Verification items for this drawing (mm, ordinates from the low corner). Coordinates: 2 decimals unless noted, no trailing zeros. Write each loop counter-clockwise with the first axis right and the second up, starting at its lowest first coordinate (ties: lowest second). Pieces come first, ordered by that corner, then holes. Notation, with made-up numbers: M 6,50.5 L 33,50.5 A32 ccw 33,78.5 Z; hole C -24,56.5 d6. An arc over 180 degrees is marked long. Put each result on its own line as item: value. Start each with the question number.
1) Cross-section at B-B on z = 0.8. Record the cut outline in (x, y), plus the area to 3 significant figures.
2) Cross-section at D-D on x = 139.5. Record the cut outline in (y, z).
3) Cross-section at C-C on y = 164.5. Record the cut outline in (x, z).
4) Gauge pin test, flat end, axial feed: pin 1 (1 mm diameter, centred on x = 141, z = 2.5, fed in from -Y). Record the tip position at first contact, or that the pin passes through.
5) Scan lines: line 1 along Y through (x, z) = (35, 2.3); line 2 along Y through (x, z) = (60, 0.8); line 3 along Y through (x, z) = (119, 2.1). Record each from-to range of solid material in increasing order.
6) Cross-section at A-A on x = 60. Record the cut outline in (y, z).
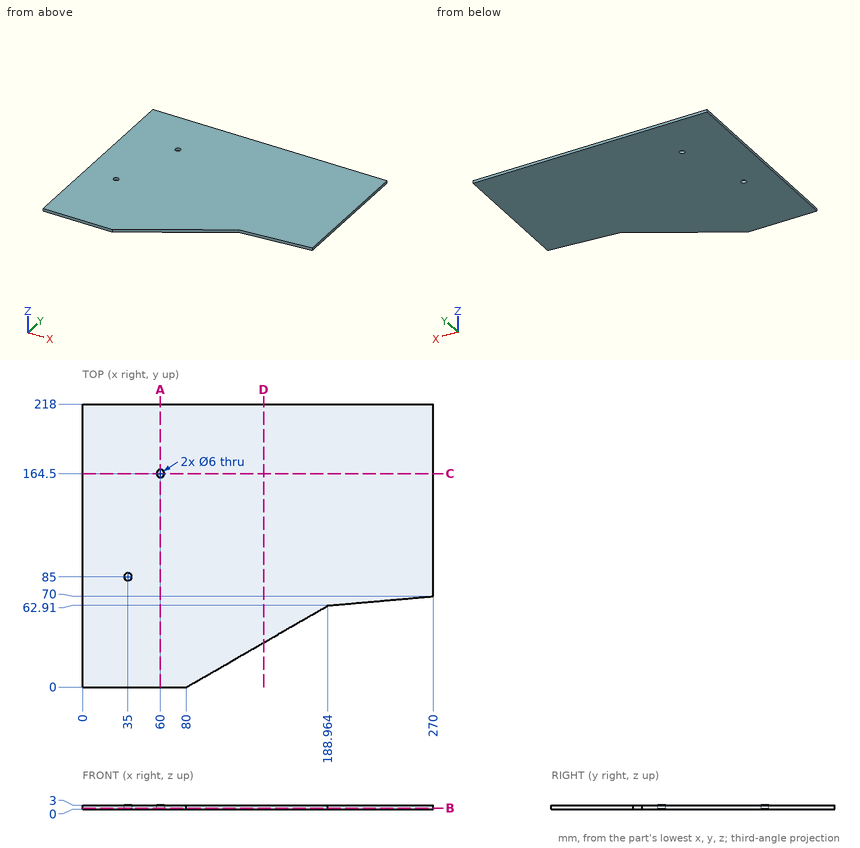
Answer key:
1. outline: M 0,0 L 80,0 L 188.96,62.91 L 270,70 L 270,218 L 0,218 Z; hole C 35,85 d6; hole C 60,164.5 d6
1. area: 50,000 mm²
2. outline: M 34.35,0 L 218,0 L 218,3 L 34.35,3 Z
3. outline: M 0,0 L 57,0 L 57,3 L 0,3 Z; M 63,0 L 270,0 L 270,3 L 63,3 Z
4. pin 1: stops at y = 34.93
5. line 1: y = 0 to 82, 88 to 218
5. line 2: y = 0 to 161.5, 167.5 to 218
5. line 3: y = 22.52 to 218
6. outline: M 0,0 L 161.5,0 L 161.5,3 L 0,3 Z; M 167.5,0 L 218,0 L 218,3 L 167.5,3 Z
